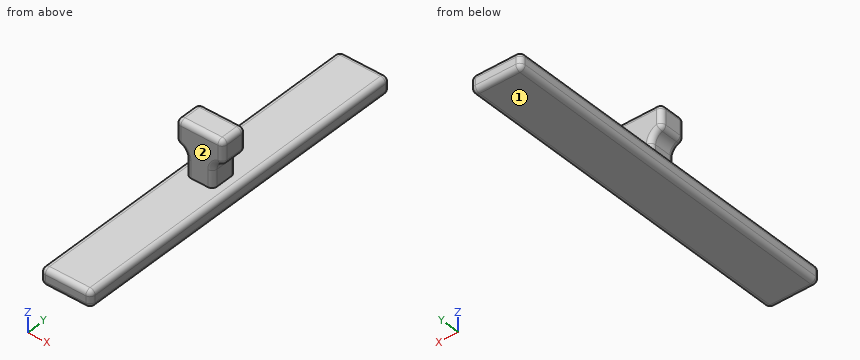
Autodesk Inventor part; units mm, degrees
ref_plane "YZ Plane" through (0, 0, 0) normal (1, 0, 0) x (0, 1, 0)
ref_plane "XZ Plane" through (0, 0, 0) normal (0, 1, 0) x (-1, 0, 0)
ref_plane "XY Plane" through (0, 0, 0) normal (0, 0, 1) x (1, 0, 0)
sketch "Sketch1" plane through (0, 0, 0) normal (0, 1, 0) x (-1, 0, 0)
  line L0 (0, 0) -> (-15, 0)
  line L1 (-15, 0) -> (-15, -5)
  line L2 (-15, -5) -> (0, -5)
  line L3 (0, -5) -> (0, 0)
  dimension "d2" = 15
  dimension "d3" = 5
extrude "Extrusion1" add sketch "Sketch1" along normal blind 105
sketch "Sketch2" plane through (0, 0, 0) normal (0, 0, 1) x (1, 0, 0)
  line L0 (3.5, 55) -> (11.5, 55)
  line L1 (11.5, 55) -> (11.5, 47)
  line L2 (11.5, 47) -> (3.5, 47)
  line L3 (3.5, 47) -> (3.5, 55)
  line L4 (0, 0) -> (15, 0)
  point P0 (7.5, 47)
  point P1 (7.5, 0)
  dimension "d6" = 8
  dimension "d7" = 8
  dimension "d8" = 55
extrude "Extrusion2" add sketch "Sketch2" along normal blind 15
sketch "Sketch3" plane through (11.5, 47, 0) normal (1, 0, 0) x (0, 0, -1)
  line L0 (0, 8) -> (-15, 8)
  line L1 (-15, 8) -> (-8, 8)
  line L2 (-8, 8) -> (-8, 0)
  line L3 (-8, 0) -> (-15, 0)
  line L4 (-15, 0) -> (-15, 8)
  point P0 (0, -47)
  dimension "d11" = 7
  dimension "d12" = 8
extrude "Extrusion3" add sketch "Sketch3" along normal blind 3
sketch "Sketch4" plane through (3.5, 47, 0) normal (-1, 0, 0) x (0, 0, 1)
  line L0 (15, 8) -> (15, 0)
  line L1 (15, 8) -> (8, 8)
  line L2 (8, 8) -> (8, 0)
  line L3 (8, 0) -> (15, 0)
  line L4 (15, 0) -> (15, 8)
  point P0 (0, -47)
  dimension "d15" = 7
  dimension "d16" = 8
extrude "Extrusion4" add sketch "Sketch4" along normal blind 3
fillet "Fillet1" radius 3 2 edges at (3.5, 51, 8) (11.5, 51, 8)
fillet "Fillet2" radius 1.5 20 edges at (14.4998, 47, 8) (14.5, 51, 8) (14.4997, 55, 8) (14.4995, 51, 8) (11.5, 55, 2.5002) (14.5, 55, 11.5) (11.5, 47, 2.5002) (3.5, 47, 2.5002) (0.5, 47, 11.5) (14.5, 47, 11.5) (7.5, 47, 15) (7.5, 55, 15) (0.5, 51, 15) (14.5, 51, 15) (0.5003, 47, 8) (0.5003, 55, 8) (0.5005, 51, 8) (0.5, 51, 8) (3.5, 55, 2.5002) (0.5, 55, 11.5)
fillet "Fillet3" radius 1.5 12 edges at (15, 52.5, 0) (0, 52.5, 0) (0, 52.5, -5) (15, 52.5, -5) (7.5, 105, 0) (15, 105, -2.5) (7.5, 105, -5) (0, 105, -2.5) (7.5, 0, -5) (0, 0, -2.5) (7.5, 0, 0) (15, 0, -2.5)
properties part number "Latch Slide" material "Steel"
Design review of the part built by this model. Coordinates are the model's own, in mm. Face numbers are marked on the shaded views. Give positions to 0.01 mm unless a question says otherwise; leave off trailing zeros. Write each loop counter-clockwise with the first axis right and the second up, starting at its lowest first coordinate (ties: lowest second). Pieces come first, ordered by that corner, then holes.
(1) Add section B-B (x = 8.5). Give the boundary of the cut face in (y, z), and give its area (3 significant figures).
Checked values:
outline: (0, -3.5) arc R1.5 ccw to (1.5, -5) - (103.5, -5) arc R1.5 ccw to (105, -3.5) - (105, -1.5) arc R1.5 ccw to (103.5, 0) - (55, 0) - (55, 13.5) arc R1.5 ccw to (53.5, 15) - (48.5, 15) arc R1.5 ccw to (47, 13.5) - (47, 0) - (1.5, 0) arc R1.5 ccw to (0, -1.5) - close
area: 642 mm2
(2) Wall thickness on line 1 along Z through (x, y) = (9, 71); line 2 along Y through (x, z) = (5.25, 12.75); line 3 along X through (y, z) = (51.5, 14.25): over which ranges is each line inside the solid? List them lowest first.
Checked values:
line 1: z = -5 to 0
line 2: y = 47 to 55
line 3: x = 0.7 to 14.3
(3) Add section A-A (z = 10.5). Give the boundary of the cut face in (x, y), and give its area (3 significant figures).
Checked values:
outline: (0.5, 48.5) arc R1.5 ccw to (2, 47) - (13, 47) arc R1.5 ccw to (14.5, 48.5) - (14.5, 53.5) arc R1.5 ccw to (13, 55) - (2, 55) arc R1.5 ccw to (0.5, 53.5) - close
area: 110 mm2
(4) Mouldability with a two-part tool opening along Z and no side actions: class the marked faces 1 and 2 as +Z half, -Z half, draft (parallel to the pull), parting line (faces both ways), or undercut.
Checked values:
face 1: -Z half
face 2: draft
(5) Clearance check with flat-ended pins moving along their axes: pin 1 Ø4 at (x, z) = (10.5, 4) entering from -Y; pin 2 Ø8 at (x, z) = (4, 4.5) entering from +Y; pin 3 Ø1.5 at (y, z) = (52, 1.5) entering from -X; pin 4 Ø10 at (y, z) = (23, 7.5) entering from +X. State where each tip first meets the part, or that it passes through.
Checked values:
pin 1: stops at y = 47
pin 2: stops at y = 55
pin 3: stops at x = 3.5
pin 4: passes through
(6) Add section C-C (y = 66). Give the boundary of the cut face in (x, z).
Checked values:
outline: (0, -3.5) arc R1.5 ccw to (1.5, -5) - (13.5, -5) arc R1.5 ccw to (15, -3.5) - (15, -1.5) arc R1.5 ccw to (13.5, 0) - (1.5, 0) arc R1.5 ccw to (0, -1.5) - close
